```python
from build123d import *

# Parameters (mm, degrees)
F0_W     = 37.6381836832
F0_H     = 53.6863617599
F1_DEPTH = 36.068
F2_W     = 33.4818195552
F2_H     = 48.4909075312
F3_DEPTH = 49.53
F4_W     = 28.1709078699
F4_H     = 8.4743649774
F5_DEPTH = 90.17
F6_R     = 4.8215246932
F7_DEPTH = 119.126


with BuildPart() as f1:
    # F0 (on Top) → F1 (new body)
    with BuildSketch(Plane.XY):
        with Locations((-18.8190918416, 26.84318088)):
            Rectangle(F0_W, F0_H)
    extrude(amount=F1_DEPTH)

    # F2 (on face) → F3 (cut)
    with BuildSketch(Plane.XY.offset(36.068)):
        with Locations((-18.8190909103, 26.9009082112)):
            Rectangle(F2_W, F2_H)
    extrude(amount=-F3_DEPTH, mode=Mode.SUBTRACT)

    # F4 (on face) → F5 (cut)
    with BuildSketch(Plane.YZ):
        with Locations((27.0163631067, 31.8308175113)):
            Rectangle(F4_W, F4_H)
    extrude(amount=-F5_DEPTH, mode=Mode.SUBTRACT)

    # F6 (on face) → F7 (cut)
    with BuildSketch(Plane.XZ):
        with Locations((-19.3963646889, 18.3572731912)):
            Circle(F6_R)
    extrude(amount=-F7_DEPTH, mode=Mode.SUBTRACT)


solid = f1.part
```
Build history of the part. All positions in model axes, mm. A direction names the side the tool comes from. Round coordinates to 2 decimals unless told otherwise and drop trailing zeros. Write each loop counter-clockwise with the first axis right and the second up, starting at its lowest first coordinate (ties: lowest second). Pieces come first, ordered by that corner, then holes. Notation, with made-up numbers: (31.5, 69) -> (50.5, 69) arc R25 cw to (50.5, 101) -> close; hole circle Ø4 at (63.5, 26.5). An arc over 180 degrees is marked (long way). Put each result on its own line as item: value.
Item 1: Tool access for faces 1 (the face through (-1, 27, 27.594)), 2 (the face through (-22, 2, 36.068)), 3 (the face through (-35.56, 27, 18)): list every direction of +Z, -Z, +X, -X, +Y, -Y with a clear straight run to the whole face (end or side of a thin tool).
Here are the results:
face 1: +Z, +X, -X
face 2: +Z, +X, -X, +Y, -Y
face 3: +Z, -Z
Item 2: Slice it at A-A, the plane z = 32. Give the cut face in (x, y), plus the area to 3 significant figures.
Here are the results:
outline: (-37.64, 0) -> (0, 0) -> (0, 12.93) -> (-2.08, 12.93) -> (-2.08, 2.66) -> (-35.56, 2.66) -> (-35.56, 12.93) -> (-37.64, 12.93) -> close; (-37.64, 41.1) -> (-35.56, 41.1) -> (-35.56, 51.15) -> (-2.08, 51.15) -> (-2.08, 41.1) -> (0, 41.1) -> (0, 53.69) -> (-37.64, 53.69) -> close
area: 280 mm^2
Item 3: Two-plate mould, pull along X, no slides. Class faces 4 (the face through (0, 26, 18)), 5 (the face through (-14.943, 52.399, 16.511)), 6 (the face through (-15, 0, 14)), 7 (the face through (-14.943, 1.309, 16.511)): pulls with the +X half, pulls with the -X half, needs draft (parallel to the pull), parting line crosses it, or undercut.
Here are the results:
face 4: pulls with the +X half
face 5: undercut
face 6: needs draft
face 7: undercut
Item 4: Slice it at C-C, the plane x = -3. Give the cut face in (y, z), plus the area to 3 significant figures.
Here are the results:
outline: (0, 0) -> (2.66, 0) -> (2.66, 36.07) -> (0, 36.07) -> close; (51.15, 0) -> (53.69, 0) -> (53.69, 36.07) -> (51.15, 36.07) -> close
area: 187 mm^2
Item 5: Slice it at B-B, the plane y = 10. Give the cut face in (x, z), plus the area to 3 significant figures.
Here are the results:
outline: (-37.64, 0) -> (-35.56, 0) -> (-35.56, 36.07) -> (-37.64, 36.07) -> close; (-2.08, 0) -> (0, 0) -> (0, 36.07) -> (-2.08, 36.07) -> close
area: 150 mm^2
Item 6: Flat gauge pin, fed straight in: P1, Ø1, axis at x = -36.5, y = 21.5, coming from the +Z side. Where does the tip first touch, or does it go through?
Here are the results:
P1: stops at z = 27.59
Item 7: Slice it at D-D, the plane z = 10.5. Give the cut face in (x, y), plus the area to 3 significant figures.
Here are the results:
outline: (-37.64, 0) -> (0, 0) -> (0, 53.69) -> (-37.64, 53.69) -> close; hole (-35.56, 2.66) -> (-2.08, 2.66) -> (-2.08, 51.15) -> (-35.56, 51.15) -> close
area: 397 mm^2
Item 8: Wall check: probe 1 along Y at (x, z) = (-13.5, 33); probe 2 along X at (y, z) = (15.5, 24). Give the ranges that are in metal, low to high. Write a range as from..to.
Here are the results:
probe 1: y = 0..2.66, 51.15..53.69
probe 2: x = -37.64..-35.56, -2.08..0
